Check sheet for the modelled part. Datum: model origin and axes. Units: mm. Round coordinates to 2 decimals unless told otherwise and drop trailing zeros. Write each loop counter-clockwise with the first axis right and the second up, starting at its lowest first coordinate (ties: lowest second). Pieces come first, ordered by that corner, then holes. Notation, with made-up numbers: (74.25, 45) - (84.25, 45) arc R30 ccw to (84.25, 69) - close; hole circle Ø3 at (21, 88). An arc over 180 degrees is marked (long way). Use one line per item in the form item = value. Start each with the question number.
1) Section check A-A (y = -8). Record the boundary of the cut face in (x, z), then the cut area to 3 significant figures.
2) Section check C-C (y = -128.5). Record the boundary of the cut face in (x, z).
3) Scan lines: probe 1 along Z at (x, y) = (0, -14); probe 2 along Y at (x, z) = (-28, 22); probe 3 along X at (y, z) = (-13, 2). Record each from-to range of solid material in increasing order.
4) Draft check along X on faces 1 (the face through (-18, -75, -29.4)), 2 (the face through (-7.008, -106.941, -31.557)), 3 (the face through (6, -13, 0)). Enter one of: +X half, -X half, draft (parallel to the pull), parting line (faces both ways), or undercut.
5) Gauge pin test, flat ends, axial feed: P1, Ø10, axis at x = -30.5, y = -30, coming from the +Z side; P2, Ø2, axis at x = -10.5, y = -25, coming from the -Z side; P3, Ø6, axis at y = -83.5, z = 27.5, coming from the -X side. Record the tip position at first contact, or that the pin passes through.
6) Section check B-B (y = -70). Record the boundary of the cut face in (x, z).
from build123d import *

# Parameters (mm, degrees)
F0_R     = 40
F1_DEPTH = 75
F2_R     = 34
F3_DEPTH = 63
F3_TAPER = 3
F4_D     = 12
F4_DEPTH = 25
F4_TIP   = 3.6051637142


with BuildPart() as f1:
    # F0 (on Front) → F1 (new body)
    with BuildSketch(Plane.XZ):
        Circle(F0_R)
    extrude(amount=F1_DEPTH)

    # F2 (on face) → F3 (join)
    with BuildSketch(Plane.XZ.offset(75)):
        Circle(F2_R)
    extrude(amount=F3_DEPTH, taper=F3_TAPER)

    # F4
    with Locations(Plane(origin=(0, 0, 0), x_dir=(1, 0, 0), z_dir=(0, 1, 0))):
        with Locations((0, 0)):
            Hole(F4_D / 2, depth=F4_DEPTH)
            with Locations((0, 0, -(F4_DEPTH + F4_TIP / 2))):  # 118° drill point
                Cone(0, F4_D / 2, F4_TIP, mode=Mode.SUBTRACT)


solid = f1.part
Results are:
q1.outline = circle Ø80 at (0, 0); hole circle Ø12 at (0, 0)
q1.area = 4,910 mm²
q2.outline = circle Ø62.39 at (0, 0)
q3.probe_1 = -40 to -6, 6 to 40
q3.probe_2 = -75 to 0
q3.probe_3 = -39.95 to -5.66, 5.66 to 39.95
q4.face_1 = draft
q4.face_2 = parting line
q4.face_3 = undercut
q5.P1 = 30.82
q5.P2 = -38.86
q5.P3 = -22.94
q6.outline = circle Ø80 at (0, 0)
